Autodesk Inventor part; units mm, degrees
ref_plane "YZ Plane" through (0, 0, 0) normal (1, 0, 0) x (0, 1, 0)
ref_plane "XZ Plane" through (0, 0, 0) normal (0, 1, 0) x (-1, 0, 0)
ref_plane "XY Plane" through (0, 0, 0) normal (0, 0, 1) x (1, 0, 0)
sketch "Sketch1" plane through (0, 0, 0) normal (0, 0, 1) x (1, 0, 0)
  line L0 (9.734, 29.9583) -> (25.484, 18.5152)
  line L1 (25.484, 18.5152) -> (31.5, 0)
  line L2 (31.5, 0) -> (25.484, -18.5152)
  line L3 (25.484, -18.5152) -> (9.734, -29.9583)
  line L4 (9.734, -29.9583) -> (-9.734, -29.9583)
  line L5 (-9.734, -29.9583) -> (-25.484, -18.5152)
  line L6 (-25.484, -18.5152) -> (-31.5, 0)
  line L7 (-31.5, 0) -> (-25.484, 18.5152)
  line L8 (-25.484, 18.5152) -> (-9.734, 29.9583)
  line L9 (-9.734, 29.9583) -> (9.734, 29.9583)
  line L10 (0, 29.9583) -> (0, 0)
  line L11 (-13.8564, 26.9632) -> (0, 18.9632)
  line L12 (0, 18.9632) -> (13.8564, 26.9632)
  line L13 (-23.3574, 16.9702) -> (-28.8713, 0)
  line L14 (-28.8713, 0) -> (-23.3574, -16.9702)
  line L15 (-23.3574, -16.9702) -> (-8.9217, -27.4583)
  line L16 (-8.9217, -27.4583) -> (8.9217, -27.4583)
  line L17 (8.9217, -27.4583) -> (23.3574, -16.9702)
  line L18 (23.3574, -16.9702) -> (28.8713, 0)
  line L19 (28.8713, 0) -> (23.3574, 16.9702)
  line L20 (8.9217, 27.4583) -> (-8.9217, 27.4583)
  line L21 (-8.9217, 27.4583) -> (-11.4864, 25.5949)
  line L22 (-12.9919, 24.5011) -> (-23.3574, 16.9702)
  line L23 (-12.9919, 24.5011) -> (0, 17.0002)
  line L24 (23.3574, 16.9702) -> (12.9919, 24.5011)
  line L25 (11.4864, 25.5949) -> (8.9217, 27.4583)
  line L26 (0, 17.0002) -> (12.9919, 24.5011)
  line L27 (0, 16.7115) -> (-12.9763, 24.2034)
  line L28 (-12.9763, 24.2034) -> (-23.1447, 16.8156)
  line L29 (-23.1447, -16.8156) -> (-8.8405, -27.2083)
  line L30 (8.8405, -27.2083) -> (23.1447, -16.8156)
  line L31 (23.1447, 16.8156) -> (12.9763, 24.2034)
  line L32 (12.9763, 24.2034) -> (0, 16.7115)
  line L33 (-23.1447, 16.8156) -> (-23.1447, -16.8156)
  line L34 (23.1447, 16.8156) -> (23.1447, -16.8156)
  line L35 (-3.35, -27.2083) -> (-3.35, -13.7083)
  line L36 (-3.35, -13.7083) -> (3.35, -13.7083)
  line L37 (3.35, -13.7083) -> (3.35, -27.2083)
  line L38 (-8.8405, -27.2083) -> (-3.35, -27.2083)
  line L39 (3.35, -27.2083) -> (8.8405, -27.2083)
  circle A0 centre (15.4447, 19.0034) radius 3
  circle A1 centre (15.4447, 19.0034) radius 1.1
  circle A2 centre (-13.15, -20.3083) radius 3
  circle A3 centre (-13.15, -20.3083) radius 1.1
  circle A4 centre (8.85, -21.7083) radius 3
  circle A5 centre (8.85, -21.7083) radius 1.1
  circle A6 centre (15.4447, 19.0034) radius 2
  circle A7 centre (-13.15, -20.3083) radius 2
  circle A8 centre (8.85, -21.7083) radius 2
  dimension "d0" = 63
  dimension "d1" = 16
  dimension "d4" = 120
  dimension "d6" = 2.5
  dimension "d7" = 1.7
  dimension "d8" = 0.25
  dimension "d11" = 6.7
  dimension "d12" = 13.5
  dimension "d13" = 0.25
  dimension "d15" = 0.25
  dimension "d16" = 0.25
  dimension "d24" = 6
  dimension "d25" = 2.2
  dimension "d26" = 6
  dimension "d27" = 2.2
  dimension "d28" = 6
  dimension "d29" = 2.2
  dimension "d30" = 5.5
  dimension "d31" = 5.5
  dimension "d32" = 9.8
  dimension "d33" = 6.9
  dimension "d36" = 5.2
  dimension "d37" = 7.7
  dimension "d38" = 4
  dimension "d39" = 4
  dimension "d40" = 4
extrude "Extrusion1" add sketch "Sketch1" along normal blind 0.8 contours L32 L31 A0 L34 L30 L39 L37 L36 L35 L38 L29 L33 L28 L27 | L31 A0 | A2 | A4 | A6 | A7 | A8 picked at (16.9034, 21.0385)
properties part number "PCB" material "FR4"
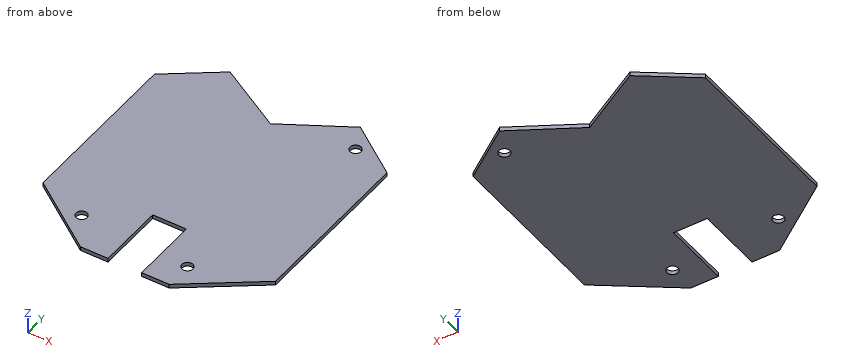
Check sheet for the modelled part. Datum: model origin and axes. Units: mm. Give positions to 0.01 mm unless a question says otherwise; leave off trailing zeros. Loops run counter-clockwise (first coordinate to the right, second up) from the corner with the lowest first, then second, coordinate; pieces in that order, holes last. Notation, with made-up numbers: M -36,-36 L 15,-36 A14 ccw 15,-27 Z; hole C 33,-24 d5. An arc over 180 degrees is marked long. Answer in a Markdown table with one row per item.
1) Cross-section at B-B (x = 2). Enter the section's corners in (y, z), plus the area to 3 significant figures.
Solutions:
| item | result |
|---|---|
| outline | M -13.71,0 L 17.87,0 L 17.87,0.8 L -13.71,0.8 Z |
| area | 25.3 mm^2 |
2) Cross-section at A-A (z = 0.45). Enter the section's corners in (x, y), plus the area to 3 significant figures.
Solutions:
| item | result |
|---|---|
| outline | M -23.14,-16.82 L -8.84,-27.21 L -3.35,-27.21 L -3.35,-13.71 L 3.35,-13.71 L 3.35,-27.21 L 8.84,-27.21 L 23.14,-16.82 L 23.14,16.82 L 12.98,24.2 L 0,16.71 L -12.98,24.2 L -23.14,16.82 Z; hole C -13.15,-20.31 d2.2; hole C 8.85,-21.71 d2.2; hole C 15.44,19 d2.2 |
| area | 1,960 mm^2 |
3) Depth check by flat-ended pin: pin 1 (2.5 mm diameter, centred on x = -13.15, y = -20.31, fed in from -Z). Enter the tip coordinate at first touch or a pass-through.
Solutions:
| item | result |
|---|---|
| pin 1 | stops at z = 0 |
4) Thickness scan on line 1 (X direction, y = -22.5, z = 0.3); line 2 (X direction, y = 18, z = 0.1); line 3 (X direction, y = -21, z = 0.7). Record the ranges inside material, lowest first.
Solutions:
| item | result |
|---|---|
| line 1 | x = -15.32 to -3.35, 3.35 to 8.09, 9.61 to 15.32 |
| line 2 | x = -21.51 to -2.23, 2.23 to 14.99, 15.9 to 21.51 |
| line 3 | x = -17.39 to -14.01, -12.29 to -3.35, 3.35 to 8.01, 9.69 to 17.39 |
5) Cross-section at C-C (x = -18). Enter the section's corners in (y, z).
Solutions:
| item | result |
|---|---|
| outline | M -20.55,0 L 20.55,0 L 20.55,0.8 L -20.55,0.8 Z |
